Source: CAD feature listing. Evaluate the final solid. Frame: model axes, mm. A direction names the side the tool comes from. Coordinates: 2 decimals unless noted, no trailing zeros. One line per item, written item: value. Start each with the question number.
Item 1: Ray query, L1, parallel to X at y = 5.75, z = 91; L2, parallel to Z at x = -12, y = 3.25; L3, parallel to X at y = 4.25, z = 17. Return the intervals inside material, ascending. Write a range as from..to.
Item 2: Set-up query: faces 3 (the flat face through (-2, 8, 47)), 4 (the flat face through (36.5, 4, 54)), 5 (the flat face through (80, 4, 86)). Return all of +Z, -Z, +X, -X, +Y, -Y with unobstructed straight access to the full face (end or side cutting, diameter ignored); none if empty.
Item 3: Cut plane A-A, the plane y = 5. State how many separate pieces and enclosed holes the cut face has, then the cut area to 3 significant figures.
Item 4: Pin query (flat end, axial travel): P1, Ø2.5, axis at x = 15, z = -28.1, coming from the +Y side; P2, Ø4, axis at y = 6.5, z = 91.5, coming from the +X side. Return the tip coordinate at first contact, or that it passes through.
Item 5: Mould query, pull axis Z, two halves, no side actions, for faces 1 (the flat face through (-115, 4, 3)), 2 (the cylindrical face through (-34.05, 3.94, 87.32)). Classes: released by +Z, released by -Z, zero draft, split by the parting line, or undercut.
```python
from build123d import *

# Parameters (mm, degrees)
SKETCH_1_W           = 230
SKETCH_1_H           = 200
EXTRUDE_1_DEPTH      = 8
SKETCH_2_R           = 1.75
SKETCH_2_R_2         = 2.2
SKETCH_2_W           = 26
SKETCH_2_H           = 44
CUT_EXTRUDE_2_DEPTH  = 8
CUT_EXTRUDE_3_DEPTH  = 8
CUT_EXTRUDE_5_DEPTH  = 8
CUT_EXTRUDE_6_DEPTH  = 8
CUT_EXTRUDE_7_DEPTH  = 8
SKETCH_2_5_W         = 35
SKETCH_2_5_H         = 90
CUT_EXTRUDE_10_DEPTH = 8
SKETCH_4_W           = 230
SKETCH_4_H           = 35
CUT_EXTRUDE_12_DEPTH = 8
FILLET_1_R           = 3


with BuildPart() as part:
    # Sketch 1 → Extrude 1 (new body)
    with BuildSketch(Plane(origin=(0, 0, 0), x_dir=(1, 0, 0), z_dir=(0, 1, 0))):
        with Locations((0, -30.464770869)):
            Rectangle(SKETCH_1_W, SKETCH_1_H)
    extrude(amount=EXTRUDE_1_DEPTH)

    # Sketch 2 → Cut-Extrude 2 (cut)
    with BuildSketch(Plane(origin=(0, 0, 0), x_dir=(1, 0, 0), z_dir=(0, 1, 0))):
        with Locations((-33.6, -116.091664289)):
            Circle(SKETCH_2_R)
        with Locations((33.6, -116.091664289)):
            Circle(SKETCH_2_R)
        with Locations((-33.6, -36.191664289)):
            Circle(SKETCH_2_R)
        with Locations((33.6, -36.191664289)):
            Circle(SKETCH_2_R)
        with Locations((-65, -69.917622991)):
            Circle(SKETCH_2_R)
        with Locations((-41, -69.917622991)):
            Circle(SKETCH_2_R)
        with Locations((-65, -99.917622991)):
            Circle(SKETCH_2_R)
        with Locations((-41, -99.917622991)):
            Circle(SKETCH_2_R)
        with Locations((-12, -40.898074934)):
            Circle(SKETCH_2_R)
        with Locations((-24.5, -40.898074934)):
            Circle(SKETCH_2_R)
        with Locations((-18.5, -24.780477191)):
            Circle(SKETCH_2_R)
        with Locations((18.5, -24.780477191)):
            Circle(SKETCH_2_R)
        with Locations((-18.5, 12.219522809)):
            Circle(SKETCH_2_R)
        with Locations((18.5, 12.219522809)):
            Circle(SKETCH_2_R)
        with Locations((-15, 4.10192507)):
            Circle(SKETCH_2_R_2)
        with Locations((-15, 28.10192507)):
            Circle(SKETCH_2_R_2)
        with Locations((15, 4.10192507)):
            Circle(SKETCH_2_R_2)
        with Locations((15, 28.10192507)):
            Circle(SKETCH_2_R_2)
        with Locations((-68.874170888, 0.466727974)):
            Rectangle(SKETCH_2_W, SKETCH_2_H)
        with BuildLine():
            Line((55.874170888, 22.466727974), (55.874170888, -21.533272026))
            Line((55.874170888, -21.533272026), (61.624170888, -21.533272026))
            Line((61.624170888, -21.533272026), (61.624170888, -23.533272026))
            ThreePointArc((61.624170888, -23.533272026), (63.874170888, -25.783272026), (66.124170888, -23.533272026))
            Line((66.124170888, -23.533272026), (66.124170888, -21.533272026))
            Line((66.124170888, -21.533272026), (71.674170888, -21.533272026))
            Line((71.674170888, -21.533272026), (71.674170888, -23.533272026))
            ThreePointArc((71.674170888, -23.533272026), (73.874170888, -25.733272026), (76.074170888, -23.533272026))
            Line((76.074170888, -23.533272026), (76.074170888, -21.533272026))
            Line((76.074170888, -21.533272026), (81.874170888, -21.533272026))
            Line((81.874170888, -21.533272026), (81.874170888, 22.466727974))
            Line((81.874170888, 22.466727974), (76.074170888, 22.466727974))
            Line((76.074170888, 22.466727974), (76.074170888, 24.466727974))
            ThreePointArc((76.074170888, 24.466727974), (73.874170888, 26.666727974), (71.674170888, 24.466727974))
            Line((71.674170888, 24.466727974), (71.674170888, 22.466727974))
            Line((71.674170888, 22.466727974), (66.124170888, 22.466727974))
            Line((66.124170888, 22.466727974), (66.124170888, 24.466727974))
            ThreePointArc((66.124170888, 24.466727974), (63.874170888, 26.716727974), (61.624170888, 24.466727974))
            Line((61.624170888, 24.466727974), (61.624170888, 22.466727974))
            Line((61.624170888, 22.466727974), (55.874170888, 22.466727974))
        make_face()
        with BuildLine():
            Line((18.5, -119.09368767), (-18.5, -119.09368767))
            ThreePointArc((-18.5, -119.09368767), (-20.5, -121.09368767), (-18.5, -123.09368767))
            Line((-18.5, -123.09368767), (18.5, -123.09368767))
            ThreePointArc((18.5, -123.09368767), (20.5, -121.09368767), (18.5, -119.09368767))
        make_face()
        with Locations((24.5, -40.898074934)):
            Circle(SKETCH_2_R)
        with Locations((12, -40.898074934)):
            Circle(SKETCH_2_R)
        with Locations((41, -69.917622991)):
            Circle(SKETCH_2_R)
        with Locations((41, -99.917622991)):
            Circle(SKETCH_2_R)
        with Locations((65, -99.917622991)):
            Circle(SKETCH_2_R)
        with Locations((65, -69.917622991)):
            Circle(SKETCH_2_R)
    extrude(amount=CUT_EXTRUDE_2_DEPTH, mode=Mode.SUBTRACT)

    # Sketch 2_3 → Cut-Extrude 3 (cut)
    with BuildSketch(Plane(origin=(0, 0, 0), x_dir=(1, 0, 0), z_dir=(0, 1, 0))):
        with BuildLine():
            Line((-71.674170888, 24.466727974), (-71.674170888, -23.533272026))
            ThreePointArc((-71.674170888, -23.533272026), (-73.874170888, -25.733272026), (-76.074170888, -23.533272026))
            Line((-76.074170888, -23.533272026), (-76.074170888, 24.466727974))
            ThreePointArc((-76.074170888, 24.466727974), (-73.874170888, 26.666727974), (-71.674170888, 24.466727974))
        make_face()
        with BuildLine():
            Line((61.624170888, 24.466727974), (61.624170888, -23.533272026))
            ThreePointArc((61.624170888, -23.533272026), (63.874170888, -25.783272026), (66.124170888, -23.533272026))
            Line((66.124170888, -23.533272026), (66.124170888, 24.466727974))
            ThreePointArc((66.124170888, 24.466727974), (63.874170888, 26.716727974), (61.624170888, 24.466727974))
        make_face()
        with BuildLine():
            Line((-61.624170888, 24.466727974), (-61.624170888, -23.533272026))
            ThreePointArc((-61.624170888, -23.533272026), (-63.874170888, -25.783272026), (-66.124170888, -23.533272026))
            Line((-66.124170888, -23.533272026), (-66.124170888, 24.466727974))
            ThreePointArc((-66.124170888, 24.466727974), (-63.874170888, 26.716727974), (-61.624170888, 24.466727974))
        make_face()
        with BuildLine():
            Line((71.674170888, 24.466727974), (71.674170888, -23.533272026))
            ThreePointArc((71.674170888, -23.533272026), (73.874170888, -25.733272026), (76.074170888, -23.533272026))
            Line((76.074170888, -23.533272026), (76.074170888, 24.466727974))
            ThreePointArc((76.074170888, 24.466727974), (73.874170888, 26.666727974), (71.674170888, 24.466727974))
        make_face()
    extrude(amount=CUT_EXTRUDE_3_DEPTH, mode=Mode.SUBTRACT)

    # Sketch 3 → Cut-Extrude 5 (cut)
    with BuildSketch(Plane(origin=(0, 0, 0), x_dir=(1, 0, 0), z_dir=(0, 1, 0))):
        with BuildLine():
            Line((-39.885757196, 10.474245388), (-39.885757196, -11.716830422))
            ThreePointArc((-39.885757196, -11.716830422), (-42.385757196, -14.216830422), (-44.885757196, -11.716830422))
            Line((-44.885757196, -11.716830422), (-44.885757196, 10.474245388))
            ThreePointArc((-44.885757196, 10.474245388), (-42.385757196, 12.974245388), (-39.885757196, 10.474245388))
        make_face()
        with BuildLine():
            Line((39.885757196, 10.474245388), (39.885757196, -11.716830422))
            ThreePointArc((39.885757196, -11.716830422), (42.385757196, -14.216830422), (44.885757196, -11.716830422))
            Line((44.885757196, -11.716830422), (44.885757196, 10.474245388))
            ThreePointArc((44.885757196, 10.474245388), (42.385757196, 12.974245388), (39.885757196, 10.474245388))
        make_face()
    extrude(amount=CUT_EXTRUDE_5_DEPTH, mode=Mode.SUBTRACT)

    # Sketch 3_5 → Cut-Extrude 6 (cut)
    with BuildSketch(Plane(origin=(0, 0, 0), x_dir=(1, 0, 0), z_dir=(0, 1, 0))):
        with BuildLine():
            Line((-36.5, -104.818717243), (-36.5, -89.818717243))
            ThreePointArc((-36.5, -89.818717243), (-34, -87.318717243), (-31.5, -89.818717243))
            Line((-31.5, -89.818717243), (-31.5, -104.818717243))
            ThreePointArc((-31.5, -104.818717243), (-34, -107.318717243), (-36.5, -104.818717243))
        make_face()
        with BuildLine():
            Line((-31.5, -46.818717243), (-31.5, -61.818717243))
            ThreePointArc((-31.5, -61.818717243), (-34, -64.318717243), (-36.5, -61.818717243))
            Line((-36.5, -61.818717243), (-36.5, -46.818717243))
            ThreePointArc((-36.5, -46.818717243), (-34, -44.318717243), (-31.5, -46.818717243))
        make_face()
        with BuildLine():
            Line((36.5, -104.818717243), (36.5, -89.818717243))
            ThreePointArc((36.5, -89.818717243), (34, -87.318717243), (31.5, -89.818717243))
            Line((31.5, -89.818717243), (31.5, -104.818717243))
            ThreePointArc((31.5, -104.818717243), (34, -107.318717243), (36.5, -104.818717243))
        make_face()
        with BuildLine():
            Line((31.5, -46.818717243), (31.5, -61.818717243))
            ThreePointArc((31.5, -61.818717243), (34, -64.318717243), (36.5, -61.818717243))
            Line((36.5, -61.818717243), (36.5, -46.818717243))
            ThreePointArc((36.5, -46.818717243), (34, -44.318717243), (31.5, -46.818717243))
        make_face()
    extrude(amount=CUT_EXTRUDE_6_DEPTH, mode=Mode.SUBTRACT)

    # Sketch 3_6 → Cut-Extrude 7 (cut)
    with BuildSketch(Plane(origin=(0, 0, 0), x_dir=(1, 0, 0), z_dir=(0, 1, 0))):
        with BuildLine():
            Line((-7.5, -31.500429428), (7.5, -31.500429428))
            ThreePointArc((7.5, -31.500429428), (9.5, -33.500429428), (7.5, -35.500429428))
            Line((7.5, -35.500429428), (-7.5, -35.500429428))
            ThreePointArc((-7.5, -35.500429428), (-9.5, -33.500429428), (-7.5, -31.500429428))
        make_face()
    extrude(amount=CUT_EXTRUDE_7_DEPTH, mode=Mode.SUBTRACT)

    # Sketch 2_5 → Cut-Extrude 10 (cut)
    with BuildSketch(Plane(origin=(0, 0, 0), x_dir=(1, 0, 0), z_dir=(0, 1, 0))):
        with Locations((-97.5, -85.464770869)):
            Rectangle(SKETCH_2_5_W, SKETCH_2_5_H)
        with Locations((97.5, -85.464770869)):
            Rectangle(SKETCH_2_5_W, SKETCH_2_5_H)
    extrude(amount=CUT_EXTRUDE_10_DEPTH, mode=Mode.SUBTRACT)

    # Sketch 4 → Cut-Extrude 12 (cut)
    with BuildSketch(Plane(origin=(0, 0, 0), x_dir=(1, 0, 0), z_dir=(0, 1, 0))):
        with Locations((0, 52.035229131)):
            Rectangle(SKETCH_4_W, SKETCH_4_H)
    extrude(amount=CUT_EXTRUDE_12_DEPTH, mode=Mode.SUBTRACT)

    # Fillet 1
    fillet_1_edges = [part.edges().sort_by_distance(p)[0] for p in [
        (-80, 4, 130.464770869),
        (-80, 4, 40.464770869),
        (-115, 4, 40.464770869),
        (115, 4, 40.464770869),
        (80, 4, 40.464770869),
        (80, 4, 130.464770869),
        (-115, 4, -34.535229131),
        (115, 4, -34.535229131),
    ]]
    fillet(fillet_1_edges, radius=FILLET_1_R)


solid = part.part
```
From the geometry:
1. L1: x = -80..-36.5, -31.5..31.5, 36.5..80
1. L2: z = -34.54..39.15, 42.65..119.09, 123.09..130.46
1. L3: x = -115..-81.87, -55.87..55.87, 81.87..115
2. face 3: +Z, -Z, +X, -X, +Y
2. face 4: +Y, -Y
2. face 5: +Z, +X, +Y, -Y
3. separate pieces: 1
3. enclosed holes: 34
3. area: 28,100 mm²
4. P1: passes through
4. P2: stops at x = 80
5. face 1: zero draft
5. face 2: undercut
